The model under review builds one solid part; all positions refer to its coordinate system, in mm. Face numbers are marked on the shaded views. A direction names the side the tool comes from. Round coordinates to 2 decimals unless told otherwise and drop trailing zeros. Order: outer loops, then holes, each group sorted by start corner. A loop starts at its lowest first (then second) coordinate and runs counter-clockwise, first axis right, second up. Notation, with made-up numbers: M 14.25,14.25 L 46.25,14.25 A15 ccw 46.25,40.25 Z; hole C 89,-26.5 d11. An arc over 180 degrees is marked long. Answer as CSV lines item,"result". Start each with the question number.
Autodesk Inventor part; units mm, degrees
ref_plane "Work Plane2" through (609.4222, 0, -20) normal (0, 0, -1) x (-1, 0, 0)
ref_plane "YZ Plane" through (0, 0, 0) normal (1, 0, 0) x (0, 1, 0)
ref_plane "XZ Plane" through (0, 0, 0) normal (0, 1, 0) x (-1, 0, 0)
sketch "Sketch1" plane through (0, 0, 0) normal (1, 0, 0) x (0, 1, 0)
  line L0 (0, 0) -> (155.1, 0)
  line L1 (155.1, 0) -> (155.1, -10)
  line L2 (0, -20) -> (0, 0)
  line L3 (155.1, -10) -> (101.6, -10)
  line L4 (101.6, -10) -> (101.6, -20)
  line L5 (101.6, -20) -> (0, -20)
  dimension "d0" = 53.5
  dimension "d1" = 155.1
  dimension "d2" = 10
  dimension "d3" = 10
  dimension "d4" = 20
extrude "Extrusion1" add sketch "Sketch1" along normal blind 584.6
ref_plane "Work Plane2" through (609.4222, 0, -20) normal (0, 0, -1) x (-1, 0, 0)
sketch "Sketch4" plane through (0, 0, 0) normal (0, 0, 1) x (1, 0, 0)
  line L0 (0, 0) -> (0, 155.1)
  line L1 (0, 0) -> (292.3032, 0)
  line L2 (0, 0) -> (584.6, 0)
  line L3 (292.3032, 50.8) -> (292.3032, 0)
  dimension "d38" = 292.3032
  dimension "d39" = 50.8
hole "Hole1" at (292.3032, 50.8, 0) direction (0, 0, -1) diameter 12.7 end through all
properties part number "SkinnySideWOpposite" material "Wood (Birch)"
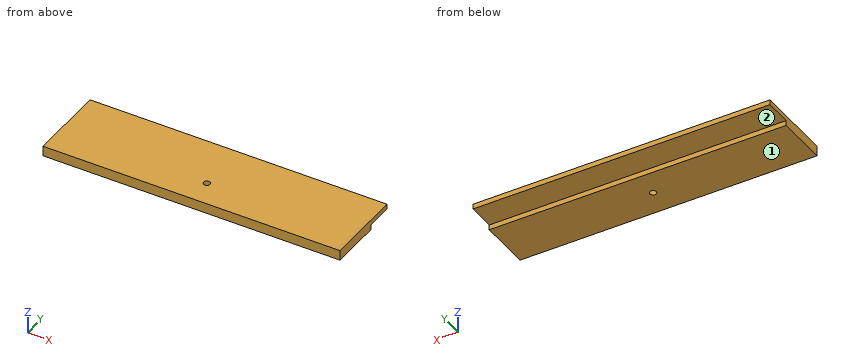
Item 1: Consider section B-B (z = -15.25). State the section outline as (x, y) points.
Item 2: Consider section C-C (x = 396.5). State the section outline as (y, z) points, and give its area (3 significant figures).
Item 3: Wall thickness on probe 1 along X at (y, z) = (50.8, -10.25); probe 2 along Y at (x, z) = (152, -17); probe 3 along Z at (x, y) = (557, 140.5): over which ranges is each line inside the solid? List them lowest first. Write a range as [from, to].
Item 4: Consider section A-A (y = 50.8). State the section outline as (x, z) points, and give its area (3 significant figures).
Item 5: Tool access review of the marked faces 1 and 2: name each direction out of +Z, -Z, +X, -X, +Y, -Y from which nothing blocks a thin tool from reaching the whole face with its end or side.
Item 6: For pin 1 (1 mm diameter, centred on x = 480, y = 123.5, fed in from -Z); pin 2 (2 mm diameter, centred on y = 60.5, z = -6, fed in from -X); pin 3 (11 mm diameter, centred on x = 351.5, z = -16.5, fed in from +Y), all flat-tipped, find the tip position at first contact; note any pin that passes through.
Reported:
1,outline,"M 0,0 L 584.6,0 L 584.6,101.6 L 0,101.6 Z; hole C 292.3,50.8 d12.7"
2,outline,"M 0,-20 L 101.6,-20 L 101.6,-10 L 155.1,-10 L 155.1,0 L 0,0 Z"
2,area,"2,570 mm²"
3,probe 1,"x = [0, 285.95], [298.65, 584.6]"
3,probe 2,"y = [0, 101.6]"
3,probe 3,"z = [-10, 0]"
4,outline,"M 0,-20 L 285.95,-20 L 285.95,0 L 0,0 Z; M 298.65,-20 L 584.6,-20 L 584.6,0 L 298.65,0 Z"
4,area,"11,400 mm²"
5,face 1,"-Z, +X, -X, +Y, -Y"
5,face 2,"-Z, +X, -X, +Y"
6,pin 1,"stops at z = -10"
6,pin 2,"stops at x = 0"
6,pin 3,"stops at y = 101.6"
